from build123d import *

# Parameters (mm, degrees)
F0_W = 12.5015752
F0_H = 17.4159876299


with BuildPart() as f1:
    # F0 (on Front) → F1 (revolve)
    with BuildSketch(Plane.XZ):
        with Locations((-6.2507876, -72.4229157223)):
            Rectangle(F0_W, F0_H)
        Polygon((-12.5015752, -63.7149219074), (0, -63.7149219074), (0, -19.4379147142), (-1.5324499691, -19.4379147142), (-3.4681754187, -23.6319862306), (-3.4681754187, -41.8600700796), (-4.9199699424, -43.9571067691), (-4.9199699424, -56.3780143857), align=None)
    revolve(axis=Axis((0, 0, -47.0220060088), (0, 0, -1)))


solid = f1.part
Could you check a few things on this model? Use its own coordinates, in mm. A direction names the side the tool comes from. Coordinates: 2 decimals unless noted, no trailing zeros. Write each loop counter-clockwise with the first axis right and the second up, starting at its lowest first coordinate (ties: lowest second). Pieces come first, ordered by that corner, then holes. Notation, with made-up numbers: (78.25, 73) - (109.25, 73) arc R15 cw to (109.25, 95) - close; hole circle Ø8 at (81, 43). An arc over 180 degrees is marked (long way). Put each result on its own line as item: value. Start each with the question number.
Q1. I'm going to push flat-ended pins straight in: P1, Ø4, axis at y = 3, z = -75, coming from the +X side; P2, Ø4, axis at x = -8.5, z = -59.5, coming from the +Y side; P3, Ø6, axis at x = 9, y = 1, coming from the +Z side. Where does each tip first touch, or does it pass through?
Q2. I want a section at C-C on z = -25.5. Write out the boundary of the cut face in (x, y).
Q3. I want a section at A-A on x = 0. Write out the boundary of the cut face in (y, z), plus the area to 3 significant figures.
Q4. Please list where these lines run through material, in increasing order: L1, parallel to Y at x = 7.5, z = -66; L2, parallel to X at y = 5.75, z = -64.5; L3, parallel to Y at x = 9, z = -64.5.
Q5. I want a section at D-D on z = -52.5. Write out the boundary of the cut face in (x, y), plus the area to 3 significant figures.
Q6. Which directions (+Z, -Z, +X, -X, +Y, -Y) give clear straight access to the entire face, cutting with the end or side of a thin tool? Please do faces 1 (the flat face through (0, 0, -19.438)), 2 (the cylindrical face through (1.067, -4.803, -50.255)).
Checks:
1. P1: x = 12.46
1. P2: y = 6.54
1. P3: z = -57.48
2. outline: circle Ø6.94 at (0, 0)
3. outline: (-12.5, -81.13) - (12.5, -81.13) - (12.5, -63.71) - (4.92, -56.38) - (4.92, -43.96) - (3.47, -41.86) - (3.47, -23.63) - (1.53, -19.44) - (-1.53, -19.44) - (-3.47, -23.63) - (-3.47, -41.86) - (-4.92, -43.96) - (-4.92, -56.38) - (-12.5, -63.71) - close
3. area: 850 mm²
4. L1: -10 to 10
4. L2: -11.1 to 11.1
4. L3: -8.68 to 8.68
5. outline: circle Ø9.84 at (0, 0)
5. area: 76.0 mm²
6. face 1: +Z, +X, -X, +Y, -Y
6. face 2: +Z
